The listing builds one solid part. Answer for the finished solid, in the listing's coordinates (mm). Face numbers are marked on the shaded views. A direction names the side the tool comes from. Coordinates: 2 decimals unless noted, no trailing zeros. Loops run counter-clockwise (first coordinate to the right, second up) from the corner with the lowest first, then second, coordinate; pieces in that order, holes last. Notation, with made-up numbers: (45, 86) - (62, 86) arc R19 cw to (62, 90) - close; hole circle Ø2 at (71.25, 2). An arc over 180 degrees is marked (long way). Put each result on its own line as item: value.
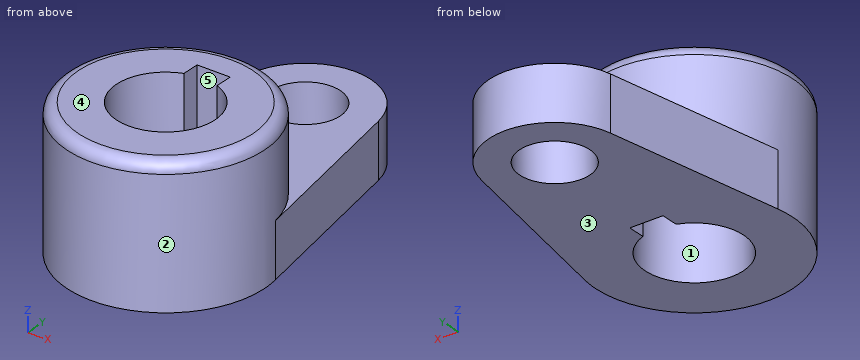
```python
from build123d import *

# Parameters (mm, degrees)
F0_R     = 28.575
F0_R_2   = 14.2875
F1_DEPTH = 40.2336
F2_R     = 10.16
F3_DEPTH = 15.7734
F4_W     = 9.652
F4_H     = 5.0815351207
F5_DEPTH = 40.2336
F6_R     = 3.302


with BuildPart() as f1:
    # F0 (on Top) → F1 (new body)
    with BuildSketch(Plane.XY):
        Circle(F0_R)
        Circle(F0_R_2, mode=Mode.SUBTRACT)
    extrude(amount=F1_DEPTH)

    # F2 (on face) → F3 (join)
    with BuildSketch(Plane(origin=(0, 0, 0), x_dir=(1, 0, 0), z_dir=(0, 0, -1))):
        with BuildLine():
            Line((-28.1265415171, -5.042646853), (-18.7510276535, -57.3367647059))
            ThreePointArc((-18.7510276535, -57.3367647059), (0, -73.025), (18.7510276535, -57.3367647059))
            Line((18.7510276535, -57.3367647059), (28.1265414639, -5.0426471501))
            ThreePointArc((28.1265414639, -5.0426471501), (-1.509e-07, -28.575), (-28.1265415171, -5.042646853))
        make_face()
        with Locations((0, -53.975)):
            Circle(F2_R, mode=Mode.SUBTRACT)
    extrude(amount=-F3_DEPTH)

    # F4 (on face) → F5 (cut, through all)
    with BuildSketch(Plane.XY.offset(40.2336)):
        with Locations((0, 15.9885324397)):
            Rectangle(F4_W, F4_H)
    extrude(amount=-F5_DEPTH, mode=Mode.SUBTRACT)

    # F6
    f6_edges = [f1.edges().sort_by_distance(p)[0] for p in [
        (-28.575, 0, 40.2336),
    ]]
    fillet(f6_edges, radius=F6_R)


solid = f1.part
```
1) Straight lines are drawn through the part: L1, parallel to Y at x = 0, z = 9 (1 decimal); L2, parallel to Y at x = -7, z = 14.5; L3, parallel to Y at x = 0, z = 17.5 (1 decimal). For each, find the intervals that lie inside material, in ascending order. Write a range as [from, to].
Found:
L1: y = [-28.6, -14.3], [18.5, 43.8], [64.1, 73]
L2: y = [-27.7, -12.46], [12.46, 46.61], [61.34, 71.69]
L3: y = [-28.6, -14.3], [18.5, 28.6]
2) The part is cut by section A-A (x = 0). Give the vertices of the cut face in (y, z) (1 decimal).
Found:
outline: (-28.6, 0) - (-14.3, 0) - (-14.3, 40.2) - (-25.3, 40.2) arc R3.3 ccw to (-28.6, 36.9) - close; (18.5, 0) - (43.8, 0) - (43.8, 15.8) - (28.6, 15.8) - (28.6, 36.9) arc R3.3 ccw to (25.3, 40.2) - (18.5, 40.2) - close; (64.1, 0) - (73, 0) - (73, 15.8) - (64.1, 15.8) - close
3) For a pull along Y with two mould halves and no side action, classify the marked faces 1, 2 and 3 as pulls with the +Y half, pulls with the -Y half, needs draft (parallel to the pull), parting line crosses it, or undercut.
Found:
face 1: undercut
face 2: parting line crosses it
face 3: needs draft
4) Each of these flat-tipped pins is pushed along its axis until it touches: pin 1 (1 mm diameter, centred on y = -7.5, z = 19.5, fed in from +X); pin 2 (4 mm diameter, centred on y = 15, z = 13.5, fed in from -X); pin 3 (8 mm diameter, centred on y = -14, z = 23, fed in from +X). Where does it stop, or does it pass through?
Found:
pin 1: stops at x = 27.7
pin 2: stops at x = -26.7
pin 3: stops at x = 26.77
5) The part is cut by section B-B (y = 0). Give the vertices of the cut face in (x, z) (1 decimal).
Found:
outline: (-28.6, 0) - (-14.3, 0) - (-14.3, 40.2) - (-25.3, 40.2) arc R3.3 ccw to (-28.6, 36.9) - close; (14.3, 0) - (28.6, 0) - (28.6, 36.9) arc R3.3 ccw to (25.3, 40.2) - (14.3, 40.2) - close
6) For the marked faces 4 and 5, determine the directions among +Z, -Z, +X, -X, +Y, -Y from which every point of the face is accessible in a straight line to the end or side of a thin tool.
Found:
face 4: +Z, +X, -X, +Y, -Y
face 5: +Z, -Z
7) The part is cut by section D-D (z = 6). State how many separate pieces and enclosed holes the cut face has, and give its area (3 significant figures).
Found:
separate pieces: 1
enclosed holes: 2
area: 3,450 mm^2
